Study the drawing (mm; zero at the part's minimum x, y, z) and answer. Round coordinates to 2 decimals unless told otherwise and drop trailing zeros. Order: outer loops, then holes, each group sorted by start corner. A loop starts at its lowest first (then second) coordinate and runs counter-clockwise, first axis right, second up. Notation, with made-up numbers: (-13.75, 68) - (-6.75, 68) arc R23 cw to (-6.75, 79) - close; hole circle Ø1 at (82.25, 5.25). An arc over 180 degrees is marked (long way). Use one line per item in the form item = value. Start each with the question number.
Q1. The part is cut by section D-D on y = 26.5. Determine the outline of the cut face in (x, z).
Q2. The part is cut by section B-B on y = 19. Determine the outline of the cut face in (x, z).
Q3. The part is cut by section A-A on x = 75. Determine the outline of the cut face in (y, z), plus the area to 3 significant figures.
Q4. The part is cut by section C-C on z = 2.25. Determine the outline of the cut face in (x, y), plus the area to 3 significant figures.
Q5. Find the intervals of material crossed by line 1 (X direction, y = 6, z = 1.7); line 2 (Y direction, x = 75, z = 2.05); line 3 (Y direction, x = 51.5, z = 1.3), in increasing order. Write a range as [from, to].
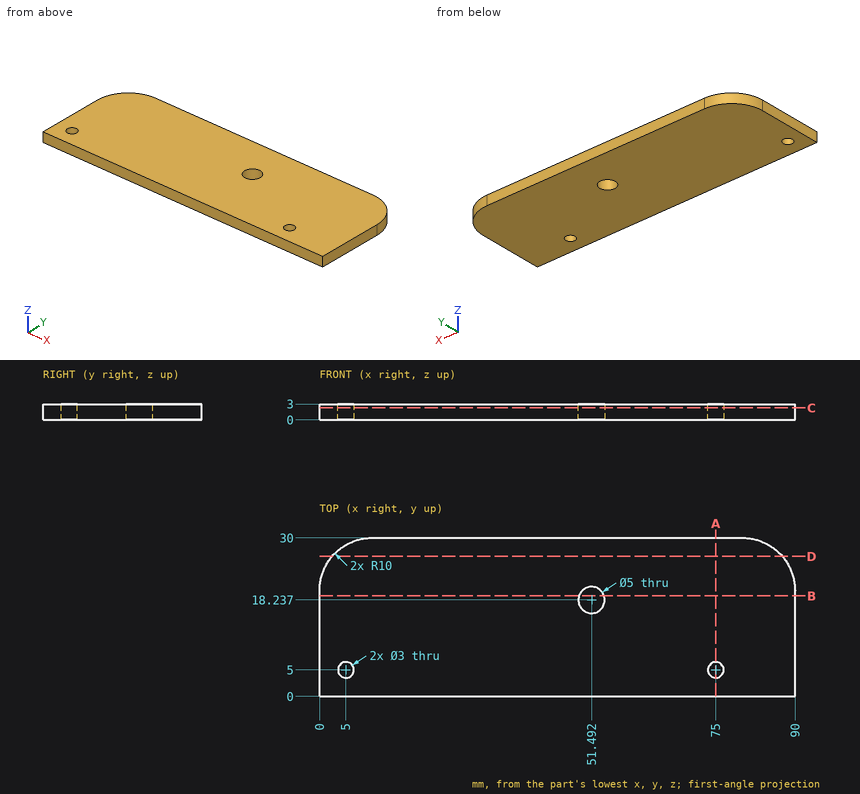
Found:
q1.outline = (2.4, 0) - (87.6, 0) - (87.6, 3) - (2.4, 3) - close
q2.outline = (0, 0) - (49.11, 0) - (49.11, 3) - (0, 3) - close; (53.87, 0) - (90, 0) - (90, 3) - (53.87, 3) - close
q3.outline = (0, 0) - (3.5, 0) - (3.5, 3) - (0, 3) - close; (6.5, 0) - (30, 0) - (30, 3) - (6.5, 3) - close
q3.area = 81.0 mm²
q4.outline = (0, 0) - (90, 0) - (90, 20) arc R10 ccw to (80, 30) - (10, 30) arc R10 ccw to (0, 20) - close; hole circle Ø3 at (5, 5); hole circle Ø5 at (51.49, 18.24); hole circle Ø3 at (75, 5)
q4.area = 2,620 mm²
q5.line_1 = [0, 3.88], [6.12, 73.88], [76.12, 90]
q5.line_2 = [0, 3.5], [6.5, 30]
q5.line_3 = [0, 15.74], [20.74, 30]
